Part model, mm, in its own coordinate system. A direction names the side the tool comes from. Give positions to 0.01 mm unless a question says otherwise; leave off trailing zeros. Order: outer loops, then holes, each group sorted by start corner. A loop starts at its lowest first (then second) coordinate and runs counter-clockwise, first axis right, second up. Notation, with made-up numbers: M 21.25,65.25 L 60.25,65.25 A26 cw 60.25,101.25 Z; hole C -37,-34.75 d1. An arc over 180 degrees is marked long. One line per question, with ' | ' between items.
```python
from build123d import *

# Parameters (mm, degrees)
F1_DEPTH = 10
F2_R     = 2.575657
F3_DEPTH = 10
F4_R     = 2


with BuildPart() as f1:
    # F0 (on Right) → F1 (new body)
    with BuildSketch(Plane.YZ):
        Polygon((-27.603682, -70), (0, -70), (27.603682, -70), (50, 0), (50, 10), (28.23673, 10), (30, 0), (20, 0), (10, 0), (11.76327, 10), (0, 10), (-11.76327, 10), (-10, 0), (-20, 0), (-30, 0), (-28.23673, 10), (-50, 10), (-50, 0), align=None)
    extrude(amount=F1_DEPTH)

    # F2 (on face) → F3 (cut, through all)
    with BuildSketch(Plane.YZ.offset(10)):
        with Locations((0, -45)):
            Circle(F2_R)
    extrude(amount=-F3_DEPTH, mode=Mode.SUBTRACT)

    # F4
    f4_edges = [f1.edges().sort_by_distance(p)[0] for p in [
        (5, -50, 10),
        (5, 50, 10),
        (10, -39.118365, 10),
        (10, 0, 10),
        (10, 39.118365, 10),
        (10, -50, 5),
        (10, -38.801841, -35),
        (10, 38.801841, -35),
        (10, 50, 5),
        (10, 0, -70),
    ]]
    fillet(f4_edges, radius=F4_R)


solid = f1.part
```
1. Drop flat-ended pins along their axis: pin 1 (1 mm diameter, centred on x = 2, z = -41.5, fed in from +Y); pin 2 (4 mm diameter, centred on y = 0, z = -45, fed in from +X); pin 3 (6 mm diameter, centred on x = 3.5, z = -38, fed in from +Y). Give the stop position or say it passes through.
Worked out:
pin 1: stops at y = 36.88 | pin 2: passes through | pin 3: stops at y = 38.8
2. Slice it at A-A on x = 1.25. Give the cut face in (y, z), then the cut area to 3 significant figures.
Worked out:
outline: M -50,0 L -27.6,-70 L 27.6,-70 L 50,0 L 50,8 A2 ccw 48,10 L 28.24,10 L 30,0 L 10,0 L 11.76,10 L -11.76,10 L -10,0 L -30,0 L -28.24,10 L -48,10 A2 ccw -50,8 Z; hole C 0,-45 d5.15 | area: 6,040 mm2
3. Slice it at C-C on z = 2.5. Give the cut face in (x, y), then the cut area to 3 significant figures.
Worked out:
outline: M 0,-50 L 8,-50 A2 ccw 10,-48 L 10,-29.56 L 0,-29.56 Z; M 0,-10.44 L 10,-10.44 L 10,10.44 L 0,10.44 Z; M 0,29.56 L 10,29.56 L 10,48 A2 ccw 8,50 L 0,50 Z | area: 616 mm2
4. Mould opens along Z. For faces 3 (the flat face through (4.9, -10.9, 5.1)), 4 (the cylindrical face through (9.43, 37.98, 9.4)), 5 (the flat face through (4, 0, -70)) say: released by +Z, released by -Z, zero draft, split by the parting line, or undercut.
Worked out:
face 3: undercut | face 4: released by +Z | face 5: released by -Z
5. Slice it at B-B on y = 0. Give the cut face in (x, z).
Worked out:
outline: M 0,-70 L 8,-70 A2 ccw 10,-68 L 10,-47.58 L 0,-47.58 Z; M 0,-42.42 L 10,-42.42 L 10,8 A2 ccw 8,10 L 0,10 Z
6. Slice it at D-D on y = -15.5. Give the cut face in (x, z), then the cut area to 3 significant figures.
Worked out:
outline: M 0,-70 L 8,-70 A2 ccw 10,-68 L 10,0 L 0,0 Z | area: 699 mm2
7. Probe L1, parallel to Y at x = 1, z = 1.5; L2, parallel to Z at x = 4.5, y = 0; L3, parallel to Z at x = 7.75, y = 23.5. List the from-to ranges inside material, lowest first. Write a range as from..to.
Worked out:
L1: y = -50..-29.74, -10.26..10.26, 29.74..50 | L2: z = -70..-47.58, -42.42..10 | L3: z = -70..0
8. Tool access for faces 1 (the cylindrical face through (4.06, 49.43, 9.4)), 2 (the flat face through (4.93, 10.87, 4.93)): list every direction of +Z, -Z, +X, -X, +Y, -Y with a clear straight run to the whole face (end or side of a thin tool).
Worked out:
face 1: +Z, +X, -X, +Y | face 2: +X, -X
